from build123d import *

# Parameters (mm, degrees)
EXTRUDE_1_DEPTH = 8
FILLET_1_R      = 0.5
FILLET_2_R      = 0.7
EXTRUDE_START   = -8
SKETCH_2_R      = 1.4
EXTRUDE_2_DEPTH = 3


with BuildPart() as part:
    # 草图1 → 凸台-拉伸1 (new body)
    with BuildSketch(Plane.XY):
        with BuildLine():
            Line((0.7, 1.212435565), (-7.960254038, 6.212435565))
            Line((-7.960254038, 6.212435565), (-10.694228634, 4.557735027))
            Line((-10.694228634, 4.557735027), (-2.9, 0.057735027))
            ThreePointArc((-2.9, 0.057735027), (-1.990417738, 0.223935223), (-1.333398647, -0.426670889))
            ThreePointArc((-1.333398647, -0.426670889), (0.878615931, -1.089969746), (0.7, 1.212435565))
        make_face()
    extrude(amount=EXTRUDE_1_DEPTH)

    # 圆角1
    fillet_1_edges = [part.edges().sort_by_distance(p)[0] for p in [
        (-7.960254038, 6.212435565, 4),
        (-2.9, 0.057735027, 4),
    ]]
    fillet(fillet_1_edges, radius=FILLET_1_R)

    # 圆角2
    fillet_2_edges = [part.edges().sort_by_distance(p)[0] for p in [
        (-10.694228634, 4.557735027, 4),
    ]]
    fillet(fillet_2_edges, radius=FILLET_2_R)

    # 草图2 → 凸台-拉伸2 (add)
    with BuildSketch(Plane(origin=(0, 0, 0), x_dir=(-1, 0, 0), z_dir=(0, 0, -1)).offset(EXTRUDE_START)):
        Circle(SKETCH_2_R)
    extrude(amount=-EXTRUDE_2_DEPTH)


solid = part.part
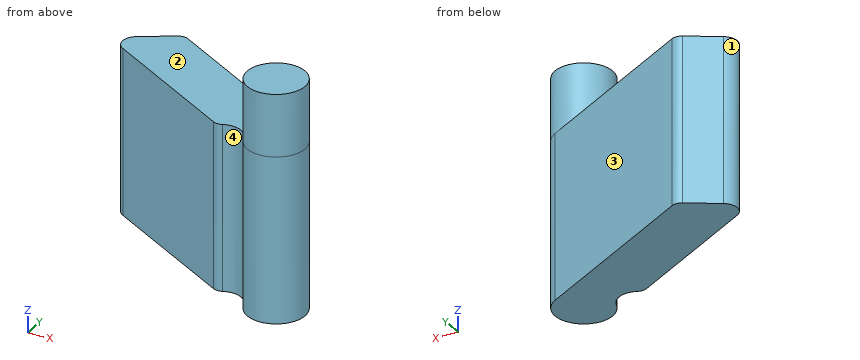
The listing builds one solid part. Answer for the finished solid, in the listing's coordinates (mm). Face numbers are marked on the shaded views. Round coordinates to 2 decimals unless told otherwise and drop trailing zeros. Order: outer loops, then holes, each group sorted by start corner. A loop starts at its lowest first (then second) coordinate and runs counter-clockwise, first axis right, second up. Notation, with made-up numbers: M -15,-25 L 2,-25 A35 cw 2,10 Z; hole C 48.25,83.5 d9. An arc over 180 degrees is marked long. Answer in a Markdown table with one row per item. Add a question column.
1) Consider line 1 along Z through (x, y) = (-1.5, 2); line 2 along X through (y, z) = (0, 8.75); line 3 along X through (y, z) = (2.75, 6.5). Determine where each line is inside the solid, lowest interval first. Write a range as from..to.
2) The part is cut by section D-D on x = -2.5. Determine the outline of the cut face in (y, z).
3) The part is cut by section C-C on y = 1. Determine the outline of the cut face in (x, z).
4) Determine the mould class of the marked faces 1, 2, 3 and 4 for opening direction X: pulls with the +X half, pulls with the -X half, needs draft (parallel to the pull), parting line crosses it, or undercut.
5) Flat-ended cylindrical pins translate along their axes: pin 1 Ø1 at (x, y) = (-7.5, 1) entering from -Z; pin 2 Ø4 at (x, y) = (-7, 3.5) entering from +Z; pin 3 Ø3 at (x, z) = (-1.5, 6.5) entering from -Y; pin 4 Ø4 at (y, z) = (2.5, 3) entering from -X. Find the tip coordinate at first contact, or state that the pin passes through.
6) The part is cut by section B-B on x = 0. Determine the outline of the cut face in (y, z), plus the area to 3 significant figures.
7) The part is cut by section A-A on z = 4.25. Determine the outline of the cut face in (x, y), plus the area to 3 significant figures.
Findings below:
| question | item | result |
|---|---|---|
| 1 | line 1 | z = 0..8 |
| 1 | line 2 | x = -1.4..1.4 |
| 1 | line 3 | x = -7.56..-1.96 |
| 2 | outline | M 0.25,0 L 3.06,0 L 3.06,8 L 0.25,8 Z |
| 3 | outline | M -4.53,0 L 0.98,0 L 0.98,11 L -0.98,11 L -0.98,8 L -4.53,8 Z |
| 4 | face 1 | pulls with the -X half |
| 4 | face 2 | needs draft |
| 4 | face 3 | pulls with the +X half |
| 4 | face 4 | undercut |
| 5 | pin 1 | passes through |
| 5 | pin 2 | stops at z = 8 |
| 5 | pin 3 | stops at y = -1.4 |
| 5 | pin 4 | stops at x = -10.02 |
| 6 | outline | M -1.4,0 L 1.62,0 L 1.62,8 L 1.4,8 L 1.4,11 L -1.4,11 Z |
| 6 | area | 32.5 mm² |
| 7 | outline | M -9.68,5.17 A0.7 ccw -9.67,3.97 L -3.15,0.2 A0.5 ccw -2.7,0.18 A1 cw -1.33,-0.43 A1.4 ccw long 0.7,1.21 L -7.7,6.06 A0.5 ccw -8.21,6.06 Z |
| 7 | area | 32.0 mm² |
